from build123d import *

# Parameters (mm, degrees)
ESBO_O1_W                = 48
ESBO_O1_H                = 46
RESSALTO_EXTRUS_O1_DEPTH = 3
ESBO_O6_W                = 3
ESBO_O6_H                = 3
RESSALTO_EXTRUS_O4_DEPTH = 3
ESBO_O2_R                = 3.55
CORTE_EXTRUS_O1_DEPTH    = 36.594943461
CORTE_EXTRUS_O2_DEPTH    = 36.594943461
PADR_OCIRCULAR1_COUNT    = 2
ESBO_O4_W                = 10
ESBO_O4_H                = 3
ESBO_O4_W_2              = 15
RESSALTO_EXTRUS_O2_DEPTH = 3
ESBO_O5_W                = 5
ESBO_O5_H                = 3
ESBO_O5_W_2              = 13
RESSALTO_EXTRUS_O3_DEPTH = 3
ESBO_O7_W                = 3
ESBO_O7_H                = 3
ESBO_O7_W_2              = 6
ESBO_O7_W_3              = 10
CORTE_EXTRUS_O3_DEPTH    = 38.603191354


with BuildPart() as part:
    # Esboço1 → Ressalto-extrusão1 (new body)
    with BuildSketch(Plane(origin=(0, 0, 0), x_dir=(1, 0, 0), z_dir=(0, 1, 0))):
        Rectangle(ESBO_O1_W, ESBO_O1_H)
    extrude(amount=RESSALTO_EXTRUS_O1_DEPTH)

    # Esboço6 → Ressalto-extrusão4 (add, through all)
    with BuildSketch(Plane(origin=(0, 0, 0), x_dir=(1, 0, 0), z_dir=(0, 1, 0))):
        with Locations((25.5, 5.5)):
            Rectangle(ESBO_O6_W, ESBO_O6_H)
    extrude(amount=RESSALTO_EXTRUS_O4_DEPTH)

    # Esboço2 → Corte-extrusão1 (cut, through all)
    with BuildSketch(Plane(origin=(0, 0, 0), x_dir=(1, 0, 0), z_dir=(0, 1, 0))):
        with Locations(Location((0, 0, 0), (0, 0, 270))):
            Circle(ESBO_O2_R)
    extrude(amount=CORTE_EXTRUS_O1_DEPTH, mode=Mode.SUBTRACT)

    # Esboço3 → Corte-extrusão2 (cut, through all)
    with BuildSketch(Plane(origin=(0, 0, 0), x_dir=(1, 0, 0), z_dir=(0, 1, 0))):
        with BuildLine():
            Line((-0.9, 10), (-0.9, 15))
            ThreePointArc((-0.9, 15), (0, 15.9), (0.9, 15))
            Line((0.9, 15), (0.9, 10))
            ThreePointArc((0.9, 10), (0, 9.1), (-0.9, 10))
        make_face()
    corte_extrus_o2 = extrude(amount=CORTE_EXTRUS_O2_DEPTH, mode=Mode.SUBTRACT)

    # PadrãoCircular1: Corte-extrusão2 ×2 about axis
    padr_ocircular1_axis = Axis((0, 0, 0), (0, 1, 0))
    for i in range(1, PADR_OCIRCULAR1_COUNT):
        add(corte_extrus_o2.rotate(padr_ocircular1_axis, i * 360 / PADR_OCIRCULAR1_COUNT), mode=Mode.SUBTRACT)

    # Esboço4 → Ressalto-extrusão2 (add, through all)
    with BuildSketch(Plane(origin=(0, 3, 0), x_dir=(1, 0, 0), z_dir=(0, 1, 0))):
        with Locations((17.7, -24.5)):
            Rectangle(ESBO_O4_W, ESBO_O4_H)
        with Locations((-14.8, -24.5)):
            Rectangle(ESBO_O4_W_2, ESBO_O4_H)
    extrude(amount=-RESSALTO_EXTRUS_O2_DEPTH)

    # Esboço5 → Ressalto-extrusão3 (add, through all)
    with BuildSketch(Plane(origin=(0, 0, 0), x_dir=(1, 0, 0), z_dir=(0, 1, 0))):
        with Locations((20, 24.5)):
            Rectangle(ESBO_O5_W, ESBO_O5_H)
        with Locations((12, 24.5)):
            Rectangle(ESBO_O5_W, ESBO_O5_H)
        with Locations((-16, 24.5)):
            Rectangle(ESBO_O5_W_2, ESBO_O5_H)
    extrude(amount=RESSALTO_EXTRUS_O3_DEPTH)

    # Esboço7 → Corte-extrusão3 (cut, through all)
    with BuildSketch(Plane(origin=(0, 0, 0), x_dir=(1, 0, 0), z_dir=(0, 1, 0))):
        with Locations((22.5, -3.3)):
            Rectangle(ESBO_O7_W, ESBO_O7_H)
        with Locations((16.5, -3.3)):
            Rectangle(ESBO_O7_W_2, ESBO_O7_H)
        with Locations((-19, -3.3)):
            Rectangle(ESBO_O7_W_3, ESBO_O7_H)
    extrude(amount=CORTE_EXTRUS_O3_DEPTH, mode=Mode.SUBTRACT)


solid = part.part
Here's how the part is built. I have some questions about the finished solid (model axes, mm). A direction names the side the tool comes from. Round coordinates to 2 decimals unless told otherwise and drop trailing zeros. Loops run counter-clockwise (first coordinate to the right, second up) from the corner with the lowest first, then second, coordinate; pieces in that order, holes last.
1. For P1, Ø1.5, axis at x = 7, y = 2.5, coming from the +Z side; P2, Ø0.9, axis at y = 1.5, z = 12.5, coming from the +X side; P3, Ø0.9, axis at y = 1.5, z = 24.5, coming from the -X side, each with a flat end and sliding along its axis, tell me the tip position at first contact or that it passes through.
Answer list:
P1: stops at z = 23
P2: stops at x = 24
P3: stops at x = -22.3
2. If we section it at C-C on z = 0: Write out the boundary of the cut face in (x, y), plus the area to 3 significant figures.
Answer list:
outline: (-24, 0) - (-3.55, 0) - (-3.55, 3) - (-24, 3) - close; (3.55, 0) - (24, 0) - (24, 3) - (3.55, 3) - close
area: 123 mm2
3. If we section it at D-D on y = 2.55: Count the separate pieces of the cut face and the enclosed holes in it, plus the area to 3 significant figures.
Answer list:
separate pieces: 1
enclosed holes: 4
area: 2,240 mm2
4. Which directions (+Z, -Z, +X, -X, +Y, -Y) give clear straight access to the entire face, cutting with the end or side of a thin tool? Please do faces 1 (the face through (23, 1, 23)), 2 (the face through (23, 1, -23)), 3 (the face through (9.5, 1, -24)).
Answer list:
face 1: +Z, +X, +Y, -Y
face 2: -Z, +X, +Y, -Y
face 3: -Z, +Y, -Y
5. If we section it at A-A on z = -11.5: Write out the boundary of the cut face in (x, y), plus the area to 3 significant figures.
Answer list:
outline: (-24, 0) - (-0.9, 0) - (-0.9, 3) - (-24, 3) - close; (0.9, 0) - (24, 0) - (24, 3) - (0.9, 3) - close
area: 139 mm2
6. We'd pull the mould along Z, two halves only. Please class faces 4 (the face through (13.5, 1, 3)), 5 (the face through (-24, 1, -10)), 6 (the face through (-23, 1, 23)), 7 (the face through (0, 1.5, -9.1)): +Z half, -Z half, draft (parallel to the pull), parting line (faces both ways), or undercut.
Answer list:
face 4: undercut
face 5: draft
face 6: +Z half
face 7: undercut
7. If we section it at B-B on x = 0: Write out the boundary of the cut face in (y, z), plus the area to 3 significant figures.
Answer list:
outline: (0, -23) - (3, -23) - (3, -15.9) - (0, -15.9) - close; (0, -9.1) - (3, -9.1) - (3, -3.55) - (0, -3.55) - close; (0, 3.55) - (3, 3.55) - (3, 9.1) - (0, 9.1) - close; (0, 15.9) - (3, 15.9) - (3, 23) - (0, 23) - close
area: 75.9 mm2
8. If I drill on line 1 along Z through (x, y) = (0, 1.35); line 2 along Z through (x, y) = (-19, 2.85); line 3 along X through (y, z) = (2.05, 0), over which ranges is the centre line in solid material (lowest first)?
Answer list:
line 1: z = -23 to -15.9, -9.1 to -3.55, 3.55 to 9.1, 15.9 to 23
line 2: z = -26 to 1.8, 4.8 to 26
line 3: x = -24 to -3.55, 3.55 to 24
